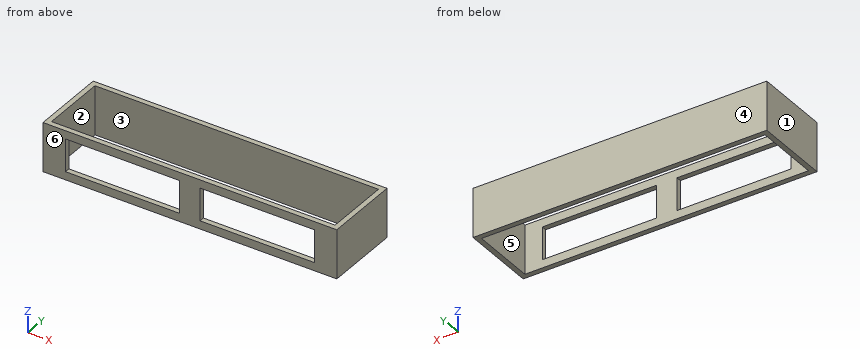
from build123d import *

# Parameters (mm, degrees)
F0_W     = 914.4
F0_H     = 15.875
F1_DEPTH = 152.4
F2_W     = 355.6
F2_H     = 101.6
F3_DEPTH = 25.4
F4_W     = 15.875
F4_H     = 152.4
F5_DEPTH = 203.2
F6_W     = 898.525
F6_H     = 152.4
F6_W_2   = 15.875
F7_DEPTH = 15.875


with BuildPart() as f1:
    # F0 (on Top) → F1 (new body)
    with BuildSketch(Plane.XY):
        with Locations((-9.282473, 39.729246)):
            Rectangle(F0_W, F0_H)
    extrude(amount=F1_DEPTH)

    # F2 (on face) → F3 (cut)
    with BuildSketch(Plane(origin=(0, 47.666746, 0), x_dir=(-1, 0, 0), z_dir=(0, 1, 0))):
        with Locations((-200.267527, 76.2)):
            Rectangle(F2_W, F2_H)
        with Locations((218.832473, 76.2)):
            Rectangle(F2_W, F2_H)
    extrude(amount=-F3_DEPTH, mode=Mode.SUBTRACT)

    # F4 (on face) → F5 (join)
    with BuildSketch(Plane(origin=(0, 47.666746, 0), x_dir=(-1, 0, 0), z_dir=(0, 1, 0))):
        with Locations((-439.980027, 76.2)):
            Rectangle(F4_W, F4_H)
        with Locations((458.544973, 76.2)):
            Rectangle(F4_W, F4_H)
    extrude(amount=F5_DEPTH)

    # F6 (on face) → F7 (join)
    with BuildSketch(Plane(origin=(0, 250.866746, 0), x_dir=(-1, 0, 0), z_dir=(0, 1, 0))):
        with Locations((17.219973, 76.2)):
            Rectangle(F6_W, F6_H)
        with Locations((-439.980027, 76.2)):
            Rectangle(F6_W_2, F6_H)
    extrude(amount=F7_DEPTH)


solid = f1.part
CAD build for the part. Positions are in the model's coordinates, mm. Face numbers are marked on the shaded views. A direction names the side the tool comes from. Coordinates: 2 decimals unless noted, no trailing zeros. Loops run counter-clockwise (first coordinate to the right, second up) from the corner with the lowest first, then second, coordinate; pieces in that order, holes last. Notation, with made-up numbers: (-21.75, 63) - (6.25, 63) arc R4 cw to (6.25, 68) - close; hole circle Ø1 at (1, 44). An arc over 180 degrees is marked (long way). Write item = value, one per line. Start each with the question number.
Q1. Cut at B-B, the plane y = 211. List the corners of the cut face in (x, z).
Q2. Drill centre lines: L1, parallel to X at y = 86, z = 77.5; L2, parallel to Y at x = -145.5, z = 133; L3, parallel to Y at x = 224, z = 76.5. Where is each one in solid material? Low to high.
Q3. Cut at D-D, the plane z = 85. List the corners of the cut face in (x, y).
Q4. Which spindle directions (+Z, -Z, +X, -X, +Y, -Y) get a long thin tool onto all of the face, cutting with end or side? Do the marked faces 5 and 6. Say none if no direction does.
Q5. Flat gauge pin, fed straight in: pin 1 Ø1.5 at (x, z) = (283.5, 32) entering from -Y. Where does the tip first touch, or does it go through?
Q6. Cut at A-A, the plane x = 388.5. List the corners of the cut face in (y, z), then the cut area to 3 significant figures.
Q7. Pull direction Y, two halves, no side cores. Call the marked faces 1, 2, 3 and 4: pulls with the +Y half, pulls with the -Y half, needs draft (parallel to the pull), parting line crosses it, or undercut.
Q8. Cut at C-C, the plane z = 11. List the corners of the cut face in (x, y).
Computed:
q1.outline = (-466.48, 0) - (-450.61, 0) - (-450.61, 152.4) - (-466.48, 152.4) - close; (432.04, 0) - (447.92, 0) - (447.92, 152.4) - (432.04, 152.4) - close
q2.L1 = -466.48 to -450.61, 432.04 to 447.92
q2.L2 = 31.79 to 47.67, 250.87 to 266.74
q2.L3 = 250.87 to 266.74
q3.outline = (-466.48, 31.79) - (-396.63, 31.79) - (-396.63, 47.67) - (-450.61, 47.67) - (-450.61, 250.87) - (432.04, 250.87) - (432.04, 47.67) - (378.07, 47.67) - (378.07, 31.79) - (447.92, 31.79) - (447.92, 266.74) - (-466.48, 266.74) - close; (-41.03, 31.79) - (22.47, 31.79) - (22.47, 47.67) - (-41.03, 47.67) - close
q4.face_5 = +Z, -Z
q4.face_6 = +Z, -Z, +X, -X, -Y
q5.pin_1 = 250.87
q6.outline = (31.79, 0) - (47.67, 0) - (47.67, 152.4) - (31.79, 152.4) - close; (250.87, 0) - (266.74, 0) - (266.74, 152.4) - (250.87, 152.4) - close
q6.area = 4,840 mm²
q7.face_1 = needs draft
q7.face_2 = undercut
q7.face_3 = undercut
q7.face_4 = pulls with the +Y half
q8.outline = (-466.48, 31.79) - (447.92, 31.79) - (447.92, 266.74) - (-466.48, 266.74) - close; hole (-450.61, 47.67) - (432.04, 47.67) - (432.04, 250.87) - (-450.61, 250.87) - close
